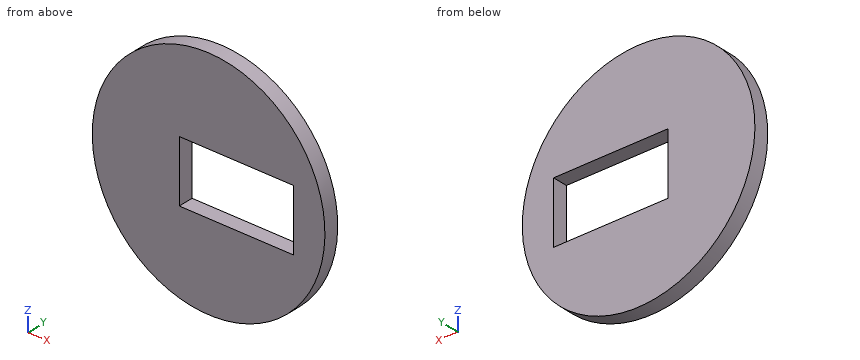
from build123d import *

# Parameters (mm, degrees)
SKETCH1_R           = 23
BOSS_EXTRUDE1_DEPTH = 3
SKETCH2_W           = 5.8
SKETCH2_H           = 6.1
SKETCH2_W_2         = 16.8
CUT_EXTRUDE1_DEPTH  = 10


with BuildPart() as part:
    # Sketch1 → Boss-Extrude1 (new body)
    with BuildSketch(Plane(origin=(0, 0, 0), x_dir=(1, 0, 0), z_dir=(0, 1, 0))):
        with Locations(Location((0, 0, 0), (0, 0, 270))):
            Circle(SKETCH1_R)
    extrude(amount=BOSS_EXTRUDE1_DEPTH)

    # Sketch2 → Cut-Extrude1 (cut)
    with BuildSketch(Plane(origin=(0, 3, 0), x_dir=(1, 0, 0), z_dir=(0, 1, 0))):
        with Locations((-2.9, 3.05)):
            Rectangle(SKETCH2_W, SKETCH2_H)
        with Locations((8.4, 3.05)):
            Rectangle(SKETCH2_W_2, SKETCH2_H)
        with Locations((8.4, -3.05)):
            Rectangle(SKETCH2_W_2, SKETCH2_H)
        with Locations((-2.9, -3.05)):
            Rectangle(SKETCH2_W, SKETCH2_H)
    extrude(amount=-CUT_EXTRUDE1_DEPTH, mode=Mode.SUBTRACT)


solid = part.part
Input: part model. Units: mm. Frame: model coordinates. Coordinates: 2 decimals unless noted, no trailing zeros. Loops run counter-clockwise (first coordinate to the right, second up) from the corner with the lowest first, then second, coordinate; pieces in that order, holes last.
Q1. Cut plane C-C (y = 1.9). Output: boundary loops of the cut face in (x, z), then the cut area to 3 significant figures.
Q2. Contact query for flat-ended pins moving along their axis: pin 1 (1.5 mm diameter, centred on x = 9.5, y = 1, fed in from +Z); pin 2 (1 mm diameter, centred on x = -9.5, y = 1.5, fed in from -Z); pin 3 (1.5 mm diameter, centred on x = -11.5, y = 0.5, fed in from -Z). Output: stop coordinate, or through.
Q3. Cut plane D-D (x = -8). Output: boundary loops of the cut face in (y, z).
Q4. Material intervals for line 1 (X direction, y = 1.85, z = 0.5); line 2 (Z direction, x = 0.5, y = 1.05); line 3 (Z direction, x = -4.5, y = 1.4), sorted ascending.
Q5. Cut plane B-B (z = 0). Output: boundary loops of the cut face in (x, y).
Q6. Cut plane A-A (x = 0). Output: boundary loops of the cut face in (y, z).
Working result:
1. outline: circle Ø46 at (0, 0); hole (-5.8, -6.1) - (16.8, -6.1) - (16.8, 6.1) - (-5.8, 6.1) - close
1. area: 1,390 mm2
2. pin 1: stops at z = 21.27
2. pin 2: stops at z = -21.17
2. pin 3: stops at z = -20.33
3. outline: (0, -21.56) - (3, -21.56) - (3, 21.56) - (0, 21.56) - close
4. line 1: x = -22.99 to -5.8, 16.8 to 22.99
4. line 2: z = -22.99 to -6.1, 6.1 to 22.99
4. line 3: z = -22.56 to -6.1, 6.1 to 22.56
5. outline: (-23, 0) - (-5.8, 0) - (-5.8, 3) - (-23, 3) - close; (16.8, 0) - (23, 0) - (23, 3) - (16.8, 3) - close
6. outline: (0, -23) - (3, -23) - (3, -6.1) - (0, -6.1) - close; (0, 6.1) - (3, 6.1) - (3, 23) - (0, 23) - close
